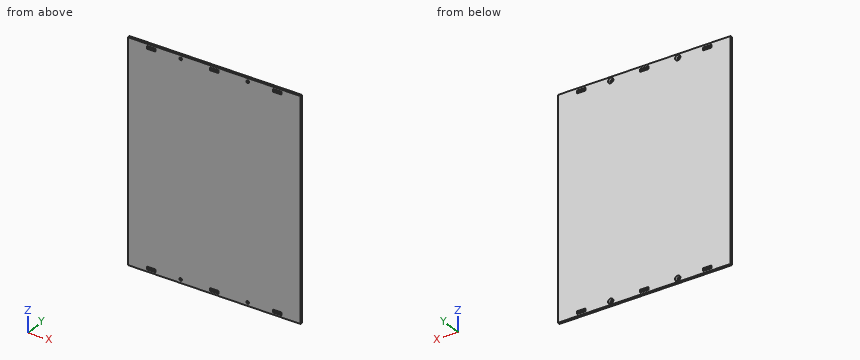
from build123d import *

# Parameters (mm, degrees)
CROQUIS1_W                                   = 220
CROQUIS1_H                                   = 280
CROQUIS1_R                                   = 1
CROQUIS1_W_2                                 = 10.5
CROQUIS1_H_2                                 = 3.5
SALIENTE_EXTRUIR1_DEPTH                      = 3
REFRENTADO_PARA_TORNILLO_TAP_N_CON_C_2_COUNT = 2
REFRENTADO_PARA_TORNILLO_TAP_N_CON_C_2_PITCH = 85.4
REFRENTADO_PARA_TORNILLO_TAP_N_CON_C_3_COUNT = 2
REFRENTADO_PARA_TORNILLO_TAP_N_CON_C_3_PITCH = 271.2
REFRENTADO_PARA_TORNILLO_TAP_N_CON_C_4_COUNT = 2
REFRENTADO_PARA_TORNILLO_TAP_N_CON_C_4_PITCH = 284.328331335


with BuildPart() as part:
    # Croquis1 → Saliente-Extruir1 (new body)
    with BuildSketch(Plane(origin=(0, 0, 0), x_dir=(1, 0, 0), z_dir=(0, 1, 0))):
        Rectangle(CROQUIS1_W, CROQUIS1_H)
        with Locations(Location((-42.7, -135.6, 0), (0, 0, 270))):
            Circle(CROQUIS1_R, mode=Mode.SUBTRACT)
        with Locations(Location((42.7, -135.6, 0), (0, 0, 90))):
            Circle(CROQUIS1_R, mode=Mode.SUBTRACT)
        with Locations(Location((42.7, 135.6, 0), (0, 0, 270))):
            Circle(CROQUIS1_R, mode=Mode.SUBTRACT)
        with Locations(Location((-42.7, 135.6, 0), (0, 0, 90))):
            Circle(CROQUIS1_R, mode=Mode.SUBTRACT)
        with Locations((-80.25, -135.6)):
            Rectangle(CROQUIS1_W_2, CROQUIS1_H_2, mode=Mode.SUBTRACT)
        with Locations((0, -135.6)):
            Rectangle(CROQUIS1_W_2, CROQUIS1_H_2, mode=Mode.SUBTRACT)
        with Locations((80.25, -135.6)):
            Rectangle(CROQUIS1_W_2, CROQUIS1_H_2, mode=Mode.SUBTRACT)
        with Locations((0, 135.6)):
            Rectangle(CROQUIS1_W_2, CROQUIS1_H_2, mode=Mode.SUBTRACT)
        with Locations((80.25, 135.6)):
            Rectangle(CROQUIS1_W_2, CROQUIS1_H_2, mode=Mode.SUBTRACT)
        with Locations((-80.25, 135.6)):
            Rectangle(CROQUIS1_W_2, CROQUIS1_H_2, mode=Mode.SUBTRACT)
    extrude(amount=SALIENTE_EXTRUIR1_DEPTH)

    # Croquis2 → Refrentado para tornillo tapón con cabeza plana de clavija de M31 (revolve, cut)
    with BuildSketch(Plane(origin=(-42.7, 3, 135.6), x_dir=(0, 0, 1), z_dir=(1, 0, 0))):
        Polygon((0, 0), (0, 3), (1.7, 3), (1.7, 1.66), (3.36, 0), align=None)
    refrentado_para_tornillo_tap_n_con_cabez = revolve(axis=Axis((-42.7, 9.35, 135.6), (0, -1, 0)), mode=Mode.SUBTRACT)

    # Refrentado para tornillo tap_n con c 2: Refrentado para tornillo tapón con cabeza plana de clavija de M31 ×2
    with Locations(*[(i * REFRENTADO_PARA_TORNILLO_TAP_N_CON_C_2_PITCH, 0, 0) for i in range(1, REFRENTADO_PARA_TORNILLO_TAP_N_CON_C_2_COUNT)]):
        add(refrentado_para_tornillo_tap_n_con_cabez, mode=Mode.SUBTRACT)

    # Refrentado para tornillo tap_n con c 3: Refrentado para tornillo tapón con cabeza plana de clavija de M31 ×2
    with Locations(*[(0, 0, -i * REFRENTADO_PARA_TORNILLO_TAP_N_CON_C_3_PITCH) for i in range(1, REFRENTADO_PARA_TORNILLO_TAP_N_CON_C_3_COUNT)]):
        add(refrentado_para_tornillo_tap_n_con_cabez, mode=Mode.SUBTRACT)

    # Refrentado para tornillo tap_n con c 4: Refrentado para tornillo tapón con cabeza plana de clavija de M31 ×2
    with Locations(*[Vector(0.3003569837690427, 0, -0.9538268618052037) * (i * REFRENTADO_PARA_TORNILLO_TAP_N_CON_C_4_PITCH) for i in range(1, REFRENTADO_PARA_TORNILLO_TAP_N_CON_C_4_COUNT)]):
        add(refrentado_para_tornillo_tap_n_con_cabez, mode=Mode.SUBTRACT)


solid = part.part
Could you check a few things on this model? Use its own coordinates, in mm. Round coordinates to 2 decimals unless told otherwise and drop trailing zeros. Loops run counter-clockwise (first coordinate to the right, second up) from the corner with the lowest first, then second, coordinate; pieces in that order, holes last. Notation, with made-up numbers: (-16.5, 54) -> (16.5, 54) arc R30 cw to (16.5, 80) -> close; hole circle Ø2 at (70.25, -32.75). An arc over 180 degrees is marked (long way). Use CSV: the item, a comma, the result in double quotes.
(1) Will this pin go through, and if not, where does the flat tip stop? pin 1 Ø2 at (x, z) = (42.7, 135.6) entering from -Y.
Return value:
pin 1,"passes through"
(2) Suppose I cut it at A-A on x = 0. Write out the boundary of the cut face in (y, z).
Return value:
outline,"(0, -140) -> (3, -140) -> (3, -137.35) -> (0, -137.35) -> close; (0, -133.85) -> (3, -133.85) -> (3, 133.85) -> (0, 133.85) -> close; (0, 137.35) -> (3, 137.35) -> (3, 140) -> (0, 140) -> close"
(3) If I drill on probe 1 along Z at (x, y) = (-1.5, 2.8); probe 2 along Z at (x, y) = (-42.7, 0.3); probe 3 along X at (y, z) = (1, -135.6), over which ranges is the centre line in solid material (lowest first)? Write a range as [from, to].
Return value:
probe 1,"z = [-140, -137.35], [-133.85, 133.85], [137.35, 140]"
probe 2,"z = [-140, -137.3], [-133.9, 133.9], [137.3, 140]"
probe 3,"x = [-110, -85.5], [-75, -44.4], [-41, -5.25], [5.25, 41], [44.4, 75], [85.5, 110]"
